The model under review builds one solid part; all positions refer to its coordinate system, in mm. Face numbers are marked on the shaded views. Give positions to 0.01 mm unless a question says otherwise; leave off trailing zeros. Write each loop counter-clockwise with the first axis right and the second up, starting at its lowest first coordinate (ties: lowest second). Pieces come first, ordered by that corner, then holes. Notation, with made-up numbers: (78, -19.75) -> (127, -19.75) arc R9 cw to (127, -2.75) -> close; hole circle Ø10 at (40.5, 29). An arc over 180 degrees is marked (long way). Use CSV: the item, a comma, the result in double quotes.
```python
from build123d import *

# Parameters (mm, degrees)
ESQUISSE1_R                  = 1.6
BOSS_EXTRU_1_DEPTH           = 8
ESQUISSE2_R                  = 1
ENL_V_MAT_EXTRU_1_DEPTH      = 8
R_P_TITION_LIN_AIRE1_COUNT   = 7
R_P_TITION_LIN_AIRE1_PITCH   = 5
ESQUISSE3_W                  = 63.02569825
ESQUISSE3_H                  = 22.447508966
ESQUISSE3_R                  = 6
ENL_V_MAT_EXTRU_2_DEPTH      = 2
ESQUISSE4_W                  = 65.150237544
ESQUISSE4_H                  = 23.585889013
ESQUISSE4_R                  = 4.65
ENL_V_MAT_EXTRU_3_DEPTH      = 1
ESQUISSE5_R                  = 2.75
ENL_V_MAT_EXTRU_4_DEPTH      = 1
CHANFREIN1_SIZE              = 1
ESQUISSE6_R                  = 4
ENL_V_MAT_EXTRU_5_DEPTH      = 5
BOSS_EXTRU_2_DEPTH           = 5
R_P_TITION_CIRCULAIRE1_COUNT = 24


with BuildPart() as part:
    # Esquisse1 → Boss.-Extru.1 (new body)
    with BuildSketch(Plane(origin=(0, 0, 0), x_dir=(1, 0, 0), z_dir=(0, 1, 0))):
        with BuildLine():
            Line((0.874233129, -7.448873501), (41.070552147, -2.731253617))
            ThreePointArc((41.070552147, -2.731253617), (43.5, 0), (41.070552147, 2.731253617))
            Line((41.070552147, 2.731253617), (0.874233129, 7.448873501))
            ThreePointArc((0.874233129, 7.448873501), (-7.5, 0), (0.874233129, -7.448873501))
        make_face()
        with Locations(Location((0, 0, 0), (0, 0, 270))):
            Circle(ESQUISSE1_R, mode=Mode.SUBTRACT)
    extrude(amount=BOSS_EXTRU_1_DEPTH)

    # Esquisse2 → Enlèv. mat.-Extru.1 (cut)
    with BuildSketch(Plane(origin=(0, 8, 0), x_dir=(1, 0, 0), z_dir=(0, 1, 0))):
        with Locations(Location((9.5, 0, 0), (0, 0, 270))):
            Circle(ESQUISSE2_R)
    enl_v_mat_extru_1 = extrude(amount=-ENL_V_MAT_EXTRU_1_DEPTH, mode=Mode.SUBTRACT)

    # Répétition linéaire1: Enlèv. mat.-Extru.1 ×7
    with Locations(*[(i * R_P_TITION_LIN_AIRE1_PITCH, 0, 0) for i in range(1, R_P_TITION_LIN_AIRE1_COUNT)]):
        add(enl_v_mat_extru_1, mode=Mode.SUBTRACT)

    # Esquisse3 → Enlèv. mat.-Extru.2 (cut)
    with BuildSketch(Plane(origin=(0, 8, 0), x_dir=(1, 0, 0), z_dir=(0, 1, 0))):
        with Locations((18.729808022, -1.006570064)):
            Rectangle(ESQUISSE3_W, ESQUISSE3_H)
        with Locations(Location((0, 0, 0), (0, 0, 270))):
            Circle(ESQUISSE3_R, mode=Mode.SUBTRACT)
    extrude(amount=-ENL_V_MAT_EXTRU_2_DEPTH, mode=Mode.SUBTRACT)

    # Esquisse4 → Enlèv. mat.-Extru.3 (cut)
    with BuildSketch(Plane.XZ):
        with Locations((19.098187779, 0.565848797)):
            Rectangle(ESQUISSE4_W, ESQUISSE4_H)
        with Locations(Location((0, 0, 0), (0, 0, 270))):
            Circle(ESQUISSE4_R, mode=Mode.SUBTRACT)
    extrude(amount=-ENL_V_MAT_EXTRU_3_DEPTH, mode=Mode.SUBTRACT)

    # Esquisse5 → Enlèv. mat.-Extru.4 (cut)
    with BuildSketch(Plane.XZ):
        with Locations(Location((0, 0, 0), (0, 0, 270))):
            Circle(ESQUISSE5_R)
    extrude(amount=-ENL_V_MAT_EXTRU_4_DEPTH, mode=Mode.SUBTRACT)

    # Chanfrein1
    chanfrein1_edges = [part.edges().sort_by_distance(p)[0] for p in [
        (0, 1, 4.65),
    ]]
    chamfer(chanfrein1_edges, length=CHANFREIN1_SIZE - 0.0001)  # a hair under: the kernel refuses the full size

    # Esquisse6 → Enlèv. mat.-Extru.5 (cut)
    with BuildSketch(Plane(origin=(0, 8, 0), x_dir=(1, 0, 0), z_dir=(0, 1, 0))):
        with Locations(Location((0, 0, 0), (0, 0, 270))):
            Circle(ESQUISSE6_R)
    extrude(amount=-ENL_V_MAT_EXTRU_5_DEPTH, mode=Mode.SUBTRACT)

    # Esquisse7 → Boss.-Extru.2 (add)
    with BuildSketch(Plane(origin=(0, 8, 0), x_dir=(1, 0, 0), z_dir=(0, 1, 0))):
        Polygon((0.3, -4), (0.139230485, -3.4), (-0.139230485, -3.4), (-0.3, -4), align=None)
    boss_extru_2 = extrude(amount=-BOSS_EXTRU_2_DEPTH)

    # Répétition circulaire1: Boss.-Extru.2 ×24 about axis
    r_p_tition_circulaire1_axis = Axis((0, 0, 0), (0, 1, 0))
    for i in range(1, R_P_TITION_CIRCULAIRE1_COUNT):
        add(boss_extru_2.rotate(r_p_tition_circulaire1_axis, i * 360 / R_P_TITION_CIRCULAIRE1_COUNT))


solid = part.part
```
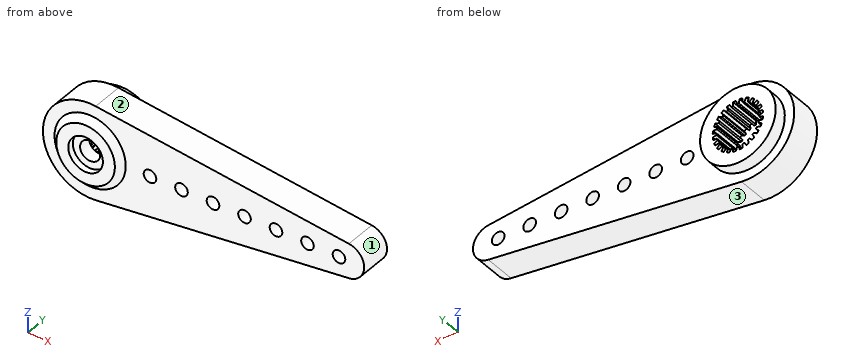
Q1. Consider section B-B (y = 3.5). State how many separate pieces and enclosed holes the cut face has, then the cut area to 3 significant figures.
Derived:
separate pieces,"1"
enclosed holes,"8"
area,"455 mm2"
Q2. Consider section C-C (x = 19.5). Write out the cut boundary in (y, z).
Derived:
outline,"(1, -5.26) -> (6, -5.26) -> (6, -1) -> (1, -1) -> close; (1, 1) -> (6, 1) -> (6, 5.26) -> (1, 5.26) -> close"
Q3. The part is to be moulded in two halves that separate along Z. For the marked faces 1, 2 and 3, say which applies: pulls with the +Z half, pulls with the -Z half, needs draft (parallel to the pull), parting line crosses it, or undercut.
Derived:
face 1,"parting line crosses it"
face 2,"pulls with the +Z half"
face 3,"pulls with the -Z half"
Q4. Insertion check: pin 1 (0.5 mm diameter, centred on x = 4, y = 6, fed in from -Z); pin 2 (2.5 mm diameter, centred on x = 34.5, z = 0, fed in from +Y); pin 3 (0.7 mm diameter, centred on x = 3.5, y = 5.5, fed in from +Z); pin 4 (2.5 mm diameter, centred on x = 0, z = 0, fed in from +Y). Each pin has a flat end and moves straight along its axis. Give the tip position at first contact, or say it passes through.
Derived:
pin 1,"stops at z = -7.11"
pin 2,"stops at y = 6"
pin 3,"stops at z = 7.18"
pin 4,"passes through"
Q5. Consider section A-A (x = 29.5). Write out the cut boundary in (y, z), then the cut area to 3 significant figures.
Derived:
outline,"(1, -4.09) -> (6, -4.09) -> (6, -1) -> (1, -1) -> close; (1, 1) -> (6, 1) -> (6, 4.09) -> (1, 4.09) -> close"
area,"30.9 mm2"
Q6. To check wall thickness, follow probe 1 along X at (y, z) = (7.75, -3); probe 2 along Y at (x, z) = (16.5, -3); probe 3 along X at (y, z) = (1.75, 1.25). State the ranges of each line that lie inside material, in increasing order.
Derived:
probe 1,"x = -5.2 to -2.59, -1.95 to -1.6, 1.6 to 1.95, 2.59 to 5.2"
probe 2,"y = 1 to 6"
probe 3,"x = -7.4 to -1, 1 to 43.2"
